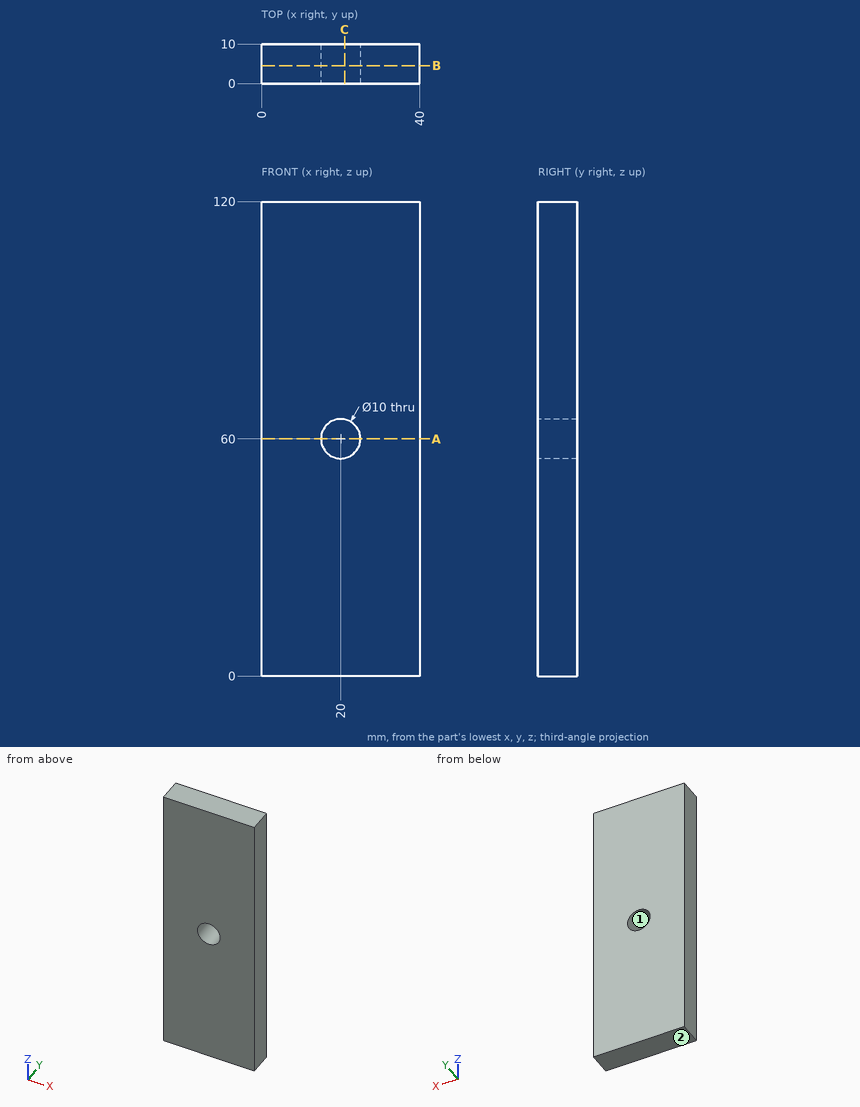
Can you work these out from the drawing? Everything is in mm from the part's minimum corner. Round coordinates to 2 decimals unless told otherwise and drop trailing zeros. Loops run counter-clockwise (first coordinate to the right, second up) from the corner with the lowest first, then second, coordinate; pieces in that order, holes last. Notation, with made-up numbers: (29.5, 72.5) - (45.5, 72.5) arc R20 cw to (45.5, 104.5) - close; hole circle Ø8 at (3, 43.25). An arc over 180 degrees is marked (long way). Answer in a Markdown table with one row per item. Add a question column.
Q1. We'd pull the mould along X, two halves only. Please class the marked faces 1 and 2: pulls with the +X half, pulls with the -X half, needs draft (parallel to the pull), parting line crosses it, or undercut.
Q2. I want a section at A-A on z = 60. List the corners of the cut face in (x, y) for me, and give its area (3 significant figures).
Q3. I want a section at C-C on x = 21. List the corners of the cut face in (y, z) for me, and give its area (3 significant figures).
Q4. I need wall thicknesses on L1, parallel to Z at x = 20, y = 7; L2, parallel to Z at x = 24, y = 8.5. Which ranges of each line are inside material? Lowest first, please.
Q5. I want a section at B-B on y = 4.5. List the corners of the cut face in (x, z) for me, and give its area (3 significant figures).
A:
| question | item | result |
|---|---|---|
| 1 | face 1 | undercut |
| 1 | face 2 | needs draft |
| 2 | outline | (0, 0) - (15, 0) - (15, 10) - (0, 10) - close; (25, 0) - (40, 0) - (40, 10) - (25, 10) - close |
| 2 | area | 300 mm^2 |
| 3 | outline | (0, 0) - (10, 0) - (10, 55.1) - (0, 55.1) - close; (0, 64.9) - (10, 64.9) - (10, 120) - (0, 120) - close |
| 3 | area | 1,100 mm^2 |
| 4 | L1 | 0 to 55, 65 to 120 |
| 4 | L2 | 0 to 57, 63 to 120 |
| 5 | outline | (0, 0) - (40, 0) - (40, 120) - (0, 120) - close; hole circle Ø10 at (20, 60) |
| 5 | area | 4,720 mm^2 |
